Can you work these out from the drawing? Everything is in mm from the part's minimum corner. Round coordinates to 2 decimals unless told otherwise and drop trailing zeros. Order: outer loops, then holes, each group sorted by start corner. A loop starts at its lowest first (then second) coordinate and runs counter-clockwise, first axis right, second up. Notation, with made-up numbers: M 27,69.25 L 75,69.25 A29 cw 75,89.25 Z; hole C 34.5,25.25 d1. An arc over 180 degrees is marked long. Write each question's results on one line, items separated by ' | '. Start each with the question number.
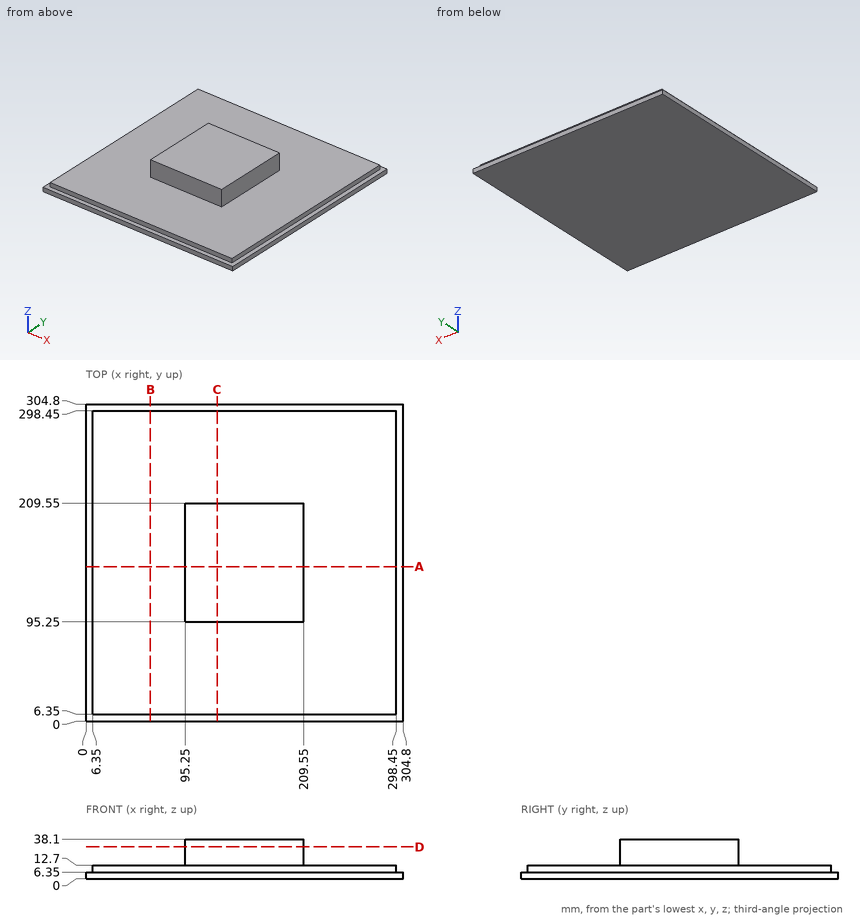
(1) I want a section at B-B on x = 62. Write out the boundary of the cut face in (y, z).
(2) Please list where these lines run through material, in increasing order: line 1 (Y direction, x = 210.5, z = 9); line 2 (Z direction, x = 180, y = 231).
(3) I want a section at D-D on z = 30.5. Write out the boundary of the cut face in (x, y), and give its area (3 significant figures).
(4) I want a section at A-A on y = 148.5. Write out the boundary of the cut face in (x, z), and give its area (3 significant figures).
(5) I'm going to push flat-ended pins straight in: pin 1 Ø1.5 at (y, z) = (273, 9.5) entering from +X; pin 2 Ø12.5 at (y, z) = (161.5, 31.5) entering from -X; pin 3 Ø10 at (x, z) = (247.5, 8.5) entering from +Y; pin 4 Ø1 at (x, y) = (215, 238.5) entering from +Z. Where does each tip first touch, or does it pass through?
Solutions:
1) outline: M 0,0 L 304.8,0 L 304.8,6.35 L 298.45,6.35 L 298.45,12.7 L 6.35,12.7 L 6.35,6.35 L 0,6.35 Z
2) line 1: 6.35 to 298.45 | line 2: 0 to 12.7
3) outline: M 95.25,95.25 L 209.55,95.25 L 209.55,209.55 L 95.25,209.55 Z | area: 13,100 mm^2
4) outline: M 0,0 L 304.8,0 L 304.8,6.35 L 298.45,6.35 L 298.45,12.7 L 209.55,12.7 L 209.55,38.1 L 95.25,38.1 L 95.25,12.7 L 6.35,12.7 L 6.35,6.35 L 0,6.35 Z | area: 6,690 mm^2
5) pin 1: x = 298.45 | pin 2: x = 95.25 | pin 3: y = 304.8 | pin 4: z = 12.7
